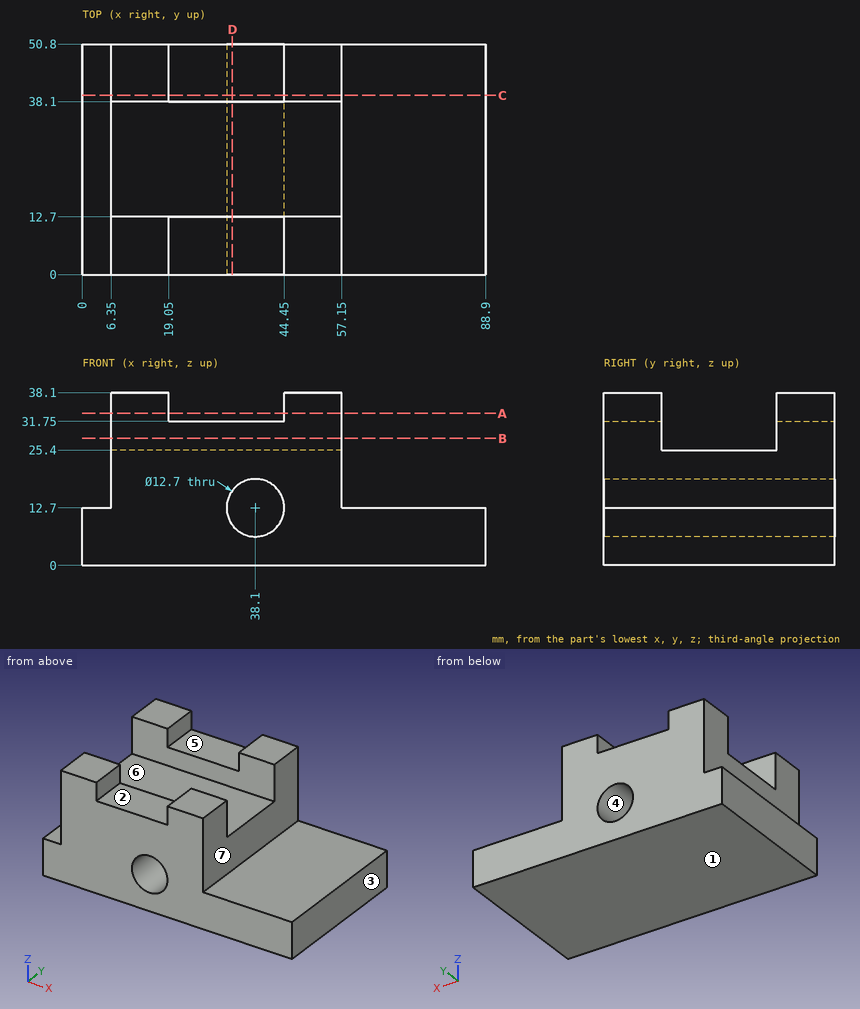
Study the drawing (mm; zero at the part's minimum x, y, z) and answer. A direction names the side the tool comes from. Give positions to 0.01 mm unless a question says otherwise; leave off trailing zeros. Order: outer loops, then holes, each group sorted by start corner. A loop starts at its lowest first (then second) coordinate and runs counter-clockwise, first axis right, second up.
1) Find section C-C on y = 39.5. Write down the section's boundary in (x, z).
Reported:
outline: (0, 0) - (88.9, 0) - (88.9, 12.7) - (57.15, 12.7) - (57.15, 38.1) - (44.45, 38.1) - (44.45, 31.75) - (19.05, 31.75) - (19.05, 38.1) - (6.35, 38.1) - (6.35, 12.7) - (0, 12.7) - close; hole circle Ø12.7 at (38.1, 12.7)
2) Find section B-B on z = 28. Write down the section's boundary in (x, y).
Reported:
outline: (6.35, 0) - (57.15, 0) - (57.15, 12.7) - (6.35, 12.7) - close; (6.35, 38.1) - (57.15, 38.1) - (57.15, 50.8) - (6.35, 50.8) - close
3) Find section A-A on z = 33.5. Write down the section's boundary in (x, y), then the cut area to 3 significant figures.
Reported:
outline: (6.35, 0) - (19.05, 0) - (19.05, 12.7) - (6.35, 12.7) - close; (6.35, 38.1) - (19.05, 38.1) - (19.05, 50.8) - (6.35, 50.8) - close; (44.45, 0) - (57.15, 0) - (57.15, 12.7) - (44.45, 12.7) - close; (44.45, 38.1) - (57.15, 38.1) - (57.15, 50.8) - (44.45, 50.8) - close
area: 645 mm2
4) Consider line 1 along Z through (x, y) = (38, 33); line 2 along Y through (x, z) = (7.5, 26); line 3 along Z through (x, y) = (8, 23). Determine where each line is inside the solid, lowest interval first.
Reported:
line 1: z = 0 to 6.35, 19.05 to 25.4
line 2: y = 0 to 12.7, 38.1 to 50.8
line 3: z = 0 to 25.4
5) Find section D-D on x = 33. Write down the section's boundary in (y, z), then the cut area to 3 significant figures.
Reported:
outline: (0, 0) - (50.8, 0) - (50.8, 8.92) - (0, 8.92) - close; (0, 16.48) - (50.8, 16.48) - (50.8, 31.75) - (38.1, 31.75) - (38.1, 25.4) - (12.7, 25.4) - (12.7, 31.75) - (0, 31.75) - close
area: 1,070 mm2
6) Given P1, Ø8, axis at y = 35.5, z = 22, coming from the -X side; P2, Ø5, axis at y = 44.5, z = 34.5, coming from the +X side; P3, Ø10, axis at x = 36.5, y = 18, coming from the +Z side, each flat-ended and moving along its own axis, determine where each tip first touches the part or whether it passes through.
Reported:
P1: stops at x = 6.35
P2: stops at x = 57.15
P3: stops at z = 25.4
7) Determine the mould class of the marked faces 1, 2, 3 and 4 for opening direction Z: pulls with the +Z half, pulls with the -Z half, needs draft (parallel to the pull), parting line crosses it, or undercut.
Reported:
face 1: pulls with the -Z half
face 2: pulls with the +Z half
face 3: needs draft
face 4: undercut
8) For the marked faces 5, 6 and 7, determine the directions among +Z, -Z, +X, -X, +Y, -Y from which every point of the face is accessible in a straight line to the end or side of a thin tool.
Reported:
face 5: +Z, +Y, -Y
face 6: +Z, +X, -X
face 7: +Z, +X, +Y, -Y
